Input: part model. Units: mm. Frame: model coordinates. A direction names the side the tool comes from. Round coordinates to 2 decimals unless told otherwise and drop trailing zeros. Loops run counter-clockwise (first coordinate to the right, second up) from the corner with the lowest first, then second, coordinate; pieces in that order, holes last. Notation, with made-up numbers: (-5.75, 16) - (28.25, 16) arc R17 ccw to (28.25, 20) - close; hole circle Ø6 at (27, 66.25). An arc over 180 degrees is marked (long way). Use CSV: the item, a comma, the result in double quotes. Start each with the question number.
1. Cut plane D-D (y = -36). Return loops of the section in (x, z).
2. Pin query (flat end, axial travel): P1, Ø2.5, axis at x = 76, y = -25, coming from the +Z side; P2, Ø5, axis at x = 33, y = -36.5, coming from the -Z side. Return the tip coordinate at first contact, or that it passes through.
3. Cut plane C-C (z = 7). Return loops of the section in (x, y).
4. Pull-direction query (Y, two-part tool) for faces 1 (the flat face through (0, -25, 15)), 2 (the cylindrical face through (0.57, -0.6, 14.79)), 3 (the flat face through (77, -15, 29)); classes: +Y half, -Y half, draft (parallel to the pull), parting line (faces both ways), or undercut.
5. Cut plane B-B (y = -28). Return loops of the section in (x, z).
6. Material intervals for probe 1 along X at (y, z) = (-20, 20.75); probe 2 along Y at (x, z) = (21, 4.5); probe 3 along Z at (x, y) = (67.5, -36.5), sorted ascending. Write a range as from..to.
7. Cut plane A-A (x = 50). Return loops of the section in (y, z), and give its area (3 significant figures).
8. Access query for faces 4 (the flat face through (2, -25, 16)), 5 (the flat face through (43, -40.825, 1)), 6 (the flat face through (3, -25, 29.918)). Directions: +Z, -Z, +X, -X, +Y, -Y. A direction counts if a zero-diameter tool reaches every point of the face in a straight line with its end or side. Return the directions, or none.
Autodesk Inventor part; units mm, degrees
ref_plane "Pracovní rovina2" through (40, -48, 0) normal (1, 0, 0) x (0, 0, -1)
ref_plane "YZ Plane" through (0, 0, 0) normal (1, 0, 0) x (0, 1, 0)
ref_plane "XZ Plane" through (0, 0, 0) normal (0, 1, 0) x (-1, 0, 0)
sketch "Náčrt3" plane through (0, 0, 0) normal (0, 0, 1) x (1, 0, 0)
  line L0 (2, 0) -> (78, 0)
  line L1 (80, -2) -> (80, -48)
  line L2 (78, -50) -> (2, -50)
  line L3 (0, -48) -> (0, -2)
  arc A0 (2, 0) -> (0, -2) centre (2, -2) ccw
  arc A1 (0, -48) -> (2, -50) centre (2, -48) ccw
  arc A2 (80, -2) -> (78, 0) centre (78, -2) ccw
  arc A3 (78, -50) -> (80, -48) centre (78, -48) ccw
  point P0 (0, 0)
  point P1 (80, -50)
  point P2 (80, 0)
  point P3 (0, -50)
  dimension "d4" = 80
  dimension "d5" = 50
  dimension "d6" = 2
extrude "Vysunutí2" add sketch "Náčrt3" along normal blind 30
shell "Skořepina1" thickness 2 removed faces 1 at (27.3333, -16.6667, 30)
sketch "Náčrt4" plane through (2, -48, 30) normal (1, 0, 0) x (0, 0, -1)
  line L0 (0.0823, 33) -> (3.0823, 33)
  line L1 (3.0823, 33) -> (3.0823, 13)
  line L2 (3.0823, 13) -> (0.0823, 13)
  line L3 (0.0823, 13) -> (0.0823, 33)
  point P0 (30, 48)
  dimension "d10" = 3
  dimension "d11" = 20
  dimension "d12" = 15
extrude "Vysunutí3" add sketch "Náčrt4" along normal blind 3
chamfer "Zkosení1" distance 2.5 angle 45 1 edges at (5, -25, 26.9177)
ref_plane "Pracovní rovina2" through (40, -48, 0) normal (1, 0, 0) x (0, 0, -1)
mirror "Zrcadlit1" about plane through (40, -48, 0) normal (1, 0, 0) of "Vysunutí3", "Zkosení1"
sketch "Náčrt5" plane through (2, -48, 2) normal (0, 0, 1) x (1, 0, 0)
  line L0 (19.0725, 36.0953) -> (62.5669, 36.0953)
  line L1 (64.5669, 34.0953) -> (64.5669, 9.1748)
  line L2 (62.5669, 7.1748) -> (19.0725, 7.1748)
  line L3 (17.0725, 9.1748) -> (17.0725, 34.0953)
  arc A0 (19.0725, 36.0953) -> (17.0725, 34.0953) centre (19.0725, 34.0953) ccw
  arc A1 (17.0725, 9.1748) -> (19.0725, 7.1748) centre (19.0725, 9.1748) ccw
  arc A2 (64.5669, 34.0953) -> (62.5669, 36.0953) centre (62.5669, 34.0953) ccw
  arc A3 (62.5669, 7.1748) -> (64.5669, 9.1748) centre (62.5669, 9.1748) ccw
  point P0 (-2, 48)
  dimension "d19" = 2
extrude "Vysunutí4" cut sketch "Náčrt5" against normal blind 3
properties part number "spodok"
Established:
1,outline,"(0, 0) - (19.07, 0) - (19.07, 2) - (2, 2) - (2, 30) - (0, 30) - close; (66.57, 0) - (80, 0) - (80, 30) - (78, 30) - (78, 2) - (66.57, 2) - close"
2,P1,"stops at z = 29.92"
2,P2,"passes through"
3,outline,"(0, -48) arc R2 ccw to (2, -50) - (78, -50) arc R2 ccw to (80, -48) - (80, -2) arc R2 ccw to (78, 0) - (2, 0) arc R2 ccw to (0, -2) - close; hole (2, -48) - (78, -48) - (78, -2) - (2, -2) - close"
4,face 1,"draft"
4,face 2,"+Y half"
4,face 3,"undercut"
5,outline,"(0, 0) - (19.07, 0) - (19.07, 2) - (2, 2) - (2, 26.92) - (2.5, 26.92) - (5, 29.42) - (5, 29.92) - (2, 29.92) - (2, 30) - (0, 30) - close; (66.57, 0) - (80, 0) - (80, 30) - (78, 30) - (78, 29.92) - (75, 29.92) - (75, 29.42) - (77.5, 26.92) - (78, 26.92) - (78, 2) - (66.57, 2) - close"
6,probe 1,"x = 0..2, 78..80"
6,probe 2,"y = -50..-48, -2..0"
6,probe 3,"z = 0..2"
7,outline,"(-50, 0) - (-40.83, 0) - (-40.83, 2) - (-48, 2) - (-48, 30) - (-50, 30) - close; (-11.9, 0) - (0, 0) - (0, 30) - (-2, 30) - (-2, 2) - (-11.9, 2) - close"
7,area,"154 mm2"
8,face 4,"none"
8,face 5,"+Z, -Z"
8,face 6,"+Z"
